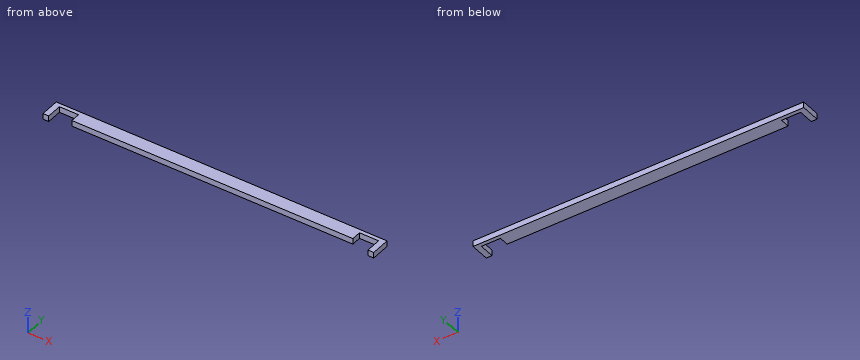
Autodesk Inventor part; units mm, degrees
ref_plane "YZ Plane" through (0, 0, 0) normal (1, 0, 0) x (0, 1, 0)
ref_plane "XZ Plane" through (0, 0, 0) normal (0, 1, 0) x (-1, 0, 0)
ref_plane "XY Plane" through (0, 0, 0) normal (0, 0, 1) x (1, 0, 0)
sketch "Sketch1" plane through (0, 0, 0) normal (0, 1, 0) x (-1, 0, 0)
  line L0 (-23.173, -32.8319) -> (-106.659, -32.8319)
  line L1 (-106.659, -32.8319) -> (-106.659, -34.3319)
  line L2 (-106.659, -34.3319) -> (-23.173, -34.3319)
  line L3 (-23.173, -34.3319) -> (-23.173, -32.8319)
  point P0 (0, 0)
  dimension "d0" = 83.486
  dimension "d1" = 1.5
extrude "Extrusion1" add sketch "Sketch1" along normal blind 3.5
ref_plane "Work Plane1" through (64.916, 0, -32.8319) normal (1, 0, 0) x (0, 0, -1)
sketch "Sketch2" plane through (23.173, 0, -32.8319) normal (0, 0, 1) x (1, 0, 0)
  line L0 (83.486, 0) -> (78.486, 0)
  line L1 (78.486, 0) -> (78.486, 2.5)
  line L2 (78.486, 2.5) -> (83.486, 2.5)
  line L3 (83.486, 2.5) -> (83.486, 0)
  point P0 (-23.173, 0)
  dimension "d4" = 2.5
  dimension "d5" = 5
extrude "Extrusion2" cut sketch "Sketch2" against normal blind 3.5
sketch "Sketch3" plane through (23.173, 3.5, -32.8319) normal (0, 0, 1) x (1, 0, 0)
  line L0 (0, 0) -> (83.486, 0)
  line L1 (83.486, 0) -> (84.986, 0)
  line L2 (84.986, 0) -> (84.986, -5)
  line L3 (84.986, -5) -> (83.486, -5)
  line L4 (83.486, -5) -> (83.486, 0)
  point P0 (-23.173, -3.5)
  dimension "d8" = 1.5
  dimension "d11" = 5
extrude "Extrusion3" add sketch "Sketch3" against normal up to surface (1.5 mm away)
mirror "Mirror1" about plane through (64.916, 0, -32.8319) normal (1, 0, 0) of "Extrusion3", "Extrusion2"
properties part number "Bar"
Input: part model. Units: mm. Frame: model coordinates. Coordinates: 2 decimals unless noted, no trailing zeros. Loops run counter-clockwise (first coordinate to the right, second up) from the corner with the lowest first, then second, coordinate; pieces in that order, holes last. Notation, with made-up numbers: M 80.25,13 L 107.25,13 A8 cw 107.25,19 Z; hole C 49,71 d9. An arc over 180 degrees is marked long. Use a Markdown table: item, result. Add a question column.
1) Line query: L1, parallel to X at y = 1.2, z = -33.2; L2, parallel to X at y = -0.3, z = -33.5; L3, parallel to Y at x = 28.5, z = -34.2. Output: solid intervals per line, ascending. Write a range as from..to.
2) Section A-A, the plane y = 0.75. Return the cut outline in (x, z).
3) Section B-B, the plane z = -33.55. Return the cut outline in (x, y).
4) Section C-C, the plane x = 79. Return the cut outline in (y, z), plus the area to 3 significant figures.
Answer below:
| question | item | result |
|---|---|---|
| 1 | L1 | 21.67..23.17, 28.17..101.66, 106.66..108.16 |
| 1 | L2 | 21.67..23.17, 106.66..108.16 |
| 1 | L3 | 0..3.5 |
| 2 | outline | M 21.67,-34.33 L 23.17,-34.33 L 23.17,-32.83 L 21.67,-32.83 Z; M 28.17,-34.33 L 101.66,-34.33 L 101.66,-32.83 L 28.17,-32.83 Z; M 106.66,-34.33 L 108.16,-34.33 L 108.16,-32.83 L 106.66,-32.83 Z |
| 3 | outline | M 21.67,-1.5 L 23.17,-1.5 L 23.17,2.5 L 28.17,2.5 L 28.17,0 L 101.66,0 L 101.66,2.5 L 106.66,2.5 L 106.66,-1.5 L 108.16,-1.5 L 108.16,3.5 L 21.67,3.5 Z |
| 4 | outline | M 0,-34.33 L 3.5,-34.33 L 3.5,-32.83 L 0,-32.83 Z |
| 4 | area | 5.25 mm2 |
